```python
from build123d import *

# Parameters (mm, degrees)
SKETCH_1_R          = 2.5
EXTRUDE_1_DEPTH     = 0.45
SKETCH_2_R          = 1.25
EXTRUDE_2_DEPTH     = 8
CHAMFER_1_SIZE      = 0.2
CUT_EXTRUDE_1_DEPTH = 0.8
FILLET_2_R          = 0.3


with BuildPart() as part:
    # 草图1 → 凸台-拉伸1 (new body, symmetric)
    with BuildSketch(Plane.XY):
        Circle(SKETCH_1_R)
    extrude(amount=EXTRUDE_1_DEPTH, both=True)

    # 草图2 → 凸台-拉伸2 (add)
    with BuildSketch(Plane(origin=(0, 0, -0.45), x_dir=(-1, 0, 0), z_dir=(0, 0, -1))):
        Circle(SKETCH_2_R)
    extrude(amount=EXTRUDE_2_DEPTH)

    # 倒角1
    chamfer_1_edges = [part.edges().sort_by_distance(p)[0] for p in [
        (1.25, 0, -8.45),
    ]]
    chamfer(chamfer_1_edges, length=CHAMFER_1_SIZE)

    # 草图3 → 切除-拉伸1 (cut)
    with BuildSketch(Plane.XY.offset(0.45)):
        Polygon((0.866025404, 0), (0.433012702, 0.75), (-0.433012702, 0.75), (-0.866025404, 0), (-0.433012702, -0.75), (0.433012702, -0.75), align=None)
    extrude(amount=-CUT_EXTRUDE_1_DEPTH, mode=Mode.SUBTRACT)

    # 圆角2
    fillet_2_edges = [part.edges().sort_by_distance(p)[0] for p in [
        (-2.5, 0, -0.45),
        (-2.5, 0, 0.45),
    ]]
    fillet(fillet_2_edges, radius=FILLET_2_R)


solid = part.part
```
Can you work these out from the model? Positions are in its coordinate system, mm. A direction names the side the tool comes from. Round coordinates to 2 decimals unless told otherwise and drop trailing zeros. Order: outer loops, then holes, each group sorted by start corner. A loop starts at its lowest first (then second) coordinate and runs counter-clockwise, first axis right, second up.
(1) On a 3-axis mill with a long thin cutter (end or side, diameter ignored), from which of +Z, -Z, +X, -X, +Y, -Y can I reach the whole of each face in a straight line? I mean faces 1 (the face through (0, 0, -8.45)), 2 (the face through (0.27, -1.22, -4.3)). Say none if no direction works.
Results are:
face 1: -Z, +X, -X, +Y, -Y
face 2: -Z
(2) If we section it at B-B (x = 0): Please give me the cut outline in (y, z).
Results are:
outline: (-2.5, -0.15) arc R0.3 ccw to (-2.2, -0.45) - (-1.25, -0.45) - (-1.25, -8.25) - (-1.05, -8.45) - (1.05, -8.45) - (1.25, -8.25) - (1.25, -0.45) - (2.2, -0.45) arc R0.3 ccw to (2.5, -0.15) - (2.5, 0.15) arc R0.3 ccw to (2.2, 0.45) - (0.75, 0.45) - (0.75, -0.35) - (-0.75, -0.35) - (-0.75, 0.45) - (-2.2, 0.45) arc R0.3 ccw to (-2.5, 0.15) - close
(3) I'm going to push flat-ended pins straight in: pin 1 (1.5 mm diameter, centred on y = -1.5, z = -2.5, fed in from +X); pin 2 (2 mm diameter, centred on x = 1.5, z = -4, fed in from +Y). Where does each tip first touch, or does it pass through?
Results are:
pin 1: stops at x = 1
pin 2: stops at y = 1.15
(4) If we section it at C-C (z = -3.5): Please give me the cut outline in (x, y), plus the area to 3 significant figures.
Results are:
outline: circle Ø2.5 at (0, 0)
area: 4.91 mm2
(5) We'd pull the mould along X, two halves only. Please class faces 3 (the face through (0, -1, 0.45)), 4 (the face through (0, 0, -0.35)), 5 (the face through (-0.54, -2.44, 0)): +X half, -X half, draft (parallel to the pull), parting line (faces both ways), or undercut.
Results are:
face 3: draft
face 4: undercut
face 5: parting line
(6) If we section it at A-A (z = 0): Please give me the cut outline in (x, y), plus the area to 3 significant figures.
Results are:
outline: circle Ø5 at (0, 0); hole (-0.87, 0) - (-0.43, -0.75) - (0.43, -0.75) - (0.87, 0) - (0.43, 0.75) - (-0.43, 0.75) - close
area: 17.7 mm2
(7) If I drill on L1, parallel to Z at x = 2, y = -0.65; L2, parallel to Z at x = -0.3, y = -0.25; L3, parallel to X at y = -0.9, z = -4.75, over which ranges is the centre line in solid material (lowest first)?
Results are:
L1: z = -0.45 to 0.45
L2: z = -8.45 to -0.35
L3: x = -0.87 to 0.87
